The model under review builds one solid part; all positions refer to its coordinate system, in mm. Round coordinates to 2 decimals unless told otherwise and drop trailing zeros. Order: outer loops, then holes, each group sorted by start corner. A loop starts at its lowest first (then second) coordinate and runs counter-clockwise, first axis right, second up.
```python
from build123d import *

# Parameters (mm, degrees)
F0_W     = 26
F0_H     = 35.5
F0_W_2   = 45
F0_H_2   = 10
F0_R     = 2
F0_R_2   = 1.05
F0_W_3   = 15
F0_R_3   = 1.1
F1_DEPTH = 2.5


with BuildPart() as f1:
    # F0 (on Top) → F1 (new body)
    with BuildSketch(Plane.XY):
        Polygon((-81.5970200658, 98.7071764616), (-96.5970200658, 98.7071764616), (-96.5970200658, -22.0728235384), (43.4029799342, -22.0728235384), (43.4029799342, 98.7071764616), (-36.5970200658, 98.7071764616), (-36.5970200658, 88.7071764616), (-35.1970200658, 88.7071764616), (-32.5970200658, 88.7071764616), (-32.5970200658, 86.1071764616), (-32.5970200658, -10.6928235384), (-32.5970200658, -13.2928235384), (-35.1970200658, -13.2928235384), (-83.9970200658, -13.2928235384), (-86.5970200658, -13.2928235384), (-86.5970200658, -10.6928235384), (-86.5970200658, 86.1071764616), (-86.5970200658, 86.5071764616), (-86.5970200658, 88.7071764616), (-84.3970200658, 88.7071764616), (-83.9970200658, 88.7071764616), (-81.5970200658, 88.7071764616), align=None)
        Polygon((-23.1610157355, -9.7928235384), (-23.1610157355, 23.2071764616), (-17.1610157355, 23.2071764616), (-17.1610157355, 33.2071764616), (-2.1610157355, 33.2071764616), (-2.1610157355, 23.2071764616), (2.8389842645, 23.2071764616), (2.8389842645, -9.7928235384), align=None, mode=Mode.SUBTRACT)
        with Locations((15.4029799342, 60.9571764616)):
            Rectangle(F0_W, F0_H, mode=Mode.SUBTRACT)
        with Locations((-59.0970200658, 93.7071764616)):
            Rectangle(F0_W_2, F0_H_2)
        Polygon((-36.5970200658, 88.7071764616), (-81.5970200658, 88.7071764616), (-83.9970200658, 88.7071764616), (-84.3970200658, 88.7071764616), (-86.5970200658, 88.7071764616), (-86.5970200658, 86.5071764616), (-86.5970200658, 86.1071764616), (-86.5970200658, -10.6928235384), (-86.5970200658, -13.2928235384), (-83.9970200658, -13.2928235384), (-35.1970200658, -13.2928235384), (-32.5970200658, -13.2928235384), (-32.5970200658, -10.6928235384), (-32.5970200658, 86.1071764616), (-32.5970200658, 88.7071764616), (-35.1970200658, 88.7071764616), align=None)
        with Locations((-83.9970200658, -10.6928235384)):
            Circle(F0_R, mode=Mode.SUBTRACT)
        with Locations((-35.1970200658, -10.6928235384)):
            Circle(F0_R, mode=Mode.SUBTRACT)
        with Locations((-83.9970200658, 86.1071764616)):
            Circle(F0_R, mode=Mode.SUBTRACT)
        with Locations((-35.1970200658, 86.1071764616)):
            Circle(F0_R, mode=Mode.SUBTRACT)
        Polygon((-17.1610157355, 23.2071764616), (-23.1610157355, 23.2071764616), (-23.1610157355, -9.7928235384), (2.8389842645, -9.7928235384), (2.8389842645, 23.2071764616), (-2.1610157355, 23.2071764616), align=None)
        with Locations((-20.3610157355, -6.9928235384)):
            Circle(F0_R_2, mode=Mode.SUBTRACT)
        with Locations((0.0389842645, -6.9928235384)):
            Circle(F0_R_2, mode=Mode.SUBTRACT)
        with Locations((-20.3610157355, 20.4071764616)):
            Circle(F0_R_2, mode=Mode.SUBTRACT)
        with Locations((0.0389842645, 20.4071764616)):
            Circle(F0_R_2, mode=Mode.SUBTRACT)
        with Locations((-9.6610157355, 28.2071764616)):
            Rectangle(F0_W_3, F0_H_2)
        with Locations((15.4029799342, 60.9571764616)):
            Rectangle(F0_W, F0_H)
        with Locations((5.0029799342, 76.1071764616)):
            Circle(F0_R_3, mode=Mode.SUBTRACT)
        with Locations((25.8029799342, 76.1071764616)):
            Circle(F0_R_3, mode=Mode.SUBTRACT)
    extrude(amount=F1_DEPTH)


solid = f1.part
```
(1) To check wall thickness, follow probe 1 along X at (y, z) = (20.5, 2.15); probe 2 along X at (y, z) = (21, 1.05); probe 3 along Y at (x, z) = (-85.5, 0.35). State the ranges of each line that lie inside material, in increasing order.
Data:
probe 1: x = -96.6 to -21.41, -19.32 to -1.01, 1.08 to 43.4
probe 2: x = -96.6 to -21.23, -19.49 to -0.83, 0.91 to 43.4
probe 3: y = -22.07 to -12.01, -9.37 to 84.79, 87.43 to 98.71
(2) Consider section A-A (x = -35). Write out the cut boundary in (y, z), and give its area (3 significant figures).
Data:
outline: (-22.07, 0) - (-12.68, 0) - (-12.68, 2.5) - (-22.07, 2.5) - close; (-8.7, 0) - (84.12, 0) - (84.12, 2.5) - (-8.7, 2.5) - close; (88.1, 0) - (98.71, 0) - (98.71, 2.5) - (88.1, 2.5) - close
area: 282 mm2
(3) Insertion check: pin 1 (2 mm diameter, centred on x = 5, y = 76.11, fed in from -Z) (1 decimal). The pin has a flat end and moves straight along its axis. Give the tip position at first contact, or say it passes through.
Data:
pin 1: passes through
(4) Draft analysis for pull direction Y (two halves, no side actions). For faces 1 (the cylindrical face through (-82.922, 87.794, 1.232)), 2 (the flat face through (-28, 39, 2.5)), state which applies: pulls with the +Y half, pulls with the -Y half, needs draft (parallel to the pull), parting line crosses it, or undercut.
Data:
face 1: undercut
face 2: needs draft
